```python
from build123d import *

# Parameters (mm, degrees)
SKETCH1_R           = 6
BOSS_EXTRUDE1_DEPTH = 110
SKETCH2_OUTSIDE_W   = 36.26
SKETCH2_OUTSIDE_H   = 36.26
SKETCH2_OUTSIDE_R   = 5
CUT_EXTRUDE1_DEPTH  = 10
SKETCH3_OUTSIDE_W   = 36.26
SKETCH3_OUTSIDE_H   = 36.26
SKETCH3_OUTSIDE_R   = 5
CUT_EXTRUDE2_DEPTH  = 10


with BuildPart() as part:
    # Sketch1 → Boss-Extrude1 (new body)
    with BuildSketch(Plane(origin=(0, 0, 0), x_dir=(0, 0, -1), z_dir=(1, 0, 0))):
        Circle(SKETCH1_R)
    extrude(amount=BOSS_EXTRUDE1_DEPTH)

    # Sketch2 outside → Cut-Extrude1 (cut)
    with BuildSketch(Plane(origin=(110, 0, 0), x_dir=(0, 0, -1), z_dir=(1, 0, 0))):
        Rectangle(SKETCH2_OUTSIDE_W, SKETCH2_OUTSIDE_H)
        Circle(SKETCH2_OUTSIDE_R, mode=Mode.SUBTRACT)
    extrude(amount=-CUT_EXTRUDE1_DEPTH, mode=Mode.SUBTRACT)

    # Sketch3 outside → Cut-Extrude2 (cut)
    with BuildSketch(Plane.ZY):
        Rectangle(SKETCH3_OUTSIDE_W, SKETCH3_OUTSIDE_H)
        with Locations(Location((0, 0, 0), (0, 0, 180))):
            Circle(SKETCH3_OUTSIDE_R, mode=Mode.SUBTRACT)
    extrude(amount=-CUT_EXTRUDE2_DEPTH, mode=Mode.SUBTRACT)


solid = part.part
```
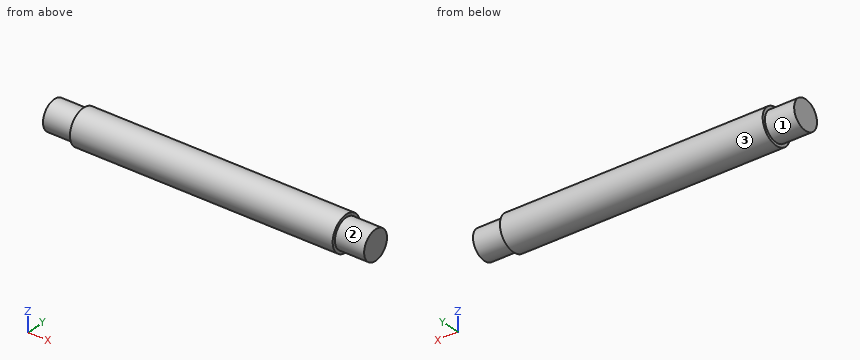
Read the model definition and answer for the solid it produces. Units are mm, in the model's axes. Face numbers are marked on the shaded views. A direction names the side the tool comes from. Coordinates: 2 decimals unless noted, no trailing zeros. Loops run counter-clockwise (first coordinate to the right, second up) from the corner with the lowest first, then second, coordinate; pieces in that order, holes last. Notation, with made-up numbers: (18, -38.5) - (31, -38.5) arc R27 ccw to (31, -21.5) - close; hole circle Ø11 at (-12.5, -21.75). An arc over 180 degrees is marked (long way). Answer in a Markdown table with one row per item.
1. Straight lines are drawn through the part: line 1 (X direction, y = -5, z = 2.75); line 2 (Z direction, x = 104, y = -0.25); line 3 (Z direction, x = 81.5, y = -2.25). For each, find the intervals that lie inside material, in ascending order.
Conclusion:
| item | result |
|---|---|
| line 1 | x = 10 to 100 |
| line 2 | z = -4.99 to 4.99 |
| line 3 | z = -5.56 to 5.56 |
2. Find section C-C, the plane x = 31.5. Write down the section's boundary in (y, z), then the cut area to 3 significant figures.
Conclusion:
| item | result |
|---|---|
| outline | circle Ø12 at (0, 0) |
| area | 113 mm² |
3. Find section A-A, the plane y = 0. Write down the section's boundary in (x, z).
Conclusion:
| item | result |
|---|---|
| outline | (0, -5) - (10, -5) - (10, -6) - (100, -6) - (100, -5) - (110, -5) - (110, 5) - (100, 5) - (100, 6) - (10, 6) - (10, 5) - (0, 5) - close |
4. Which of the six approach directions +Z, -Z, +X, -X, +Y, -Y give full straight-line access (tool end or side, diameter ignored) to the marked faces 1, 2 and 3?
Conclusion:
| item | result |
|---|---|
| face 1 | -X |
| face 2 | +X |
| face 3 | +X, -X |
5. Given pin 1 (2 mm diameter, centred on x = 27, z = 4, fed in from -Y); pin 2 (1 mm diameter, centred on x = 66.5, z = 2, fed in from -Y), each flat-ended and moving along its own axis, determine where each tip first touches the part or whether it passes through.
Conclusion:
| item | result |
|---|---|
| pin 1 | stops at y = -5.2 |
| pin 2 | stops at y = -5.81 |
